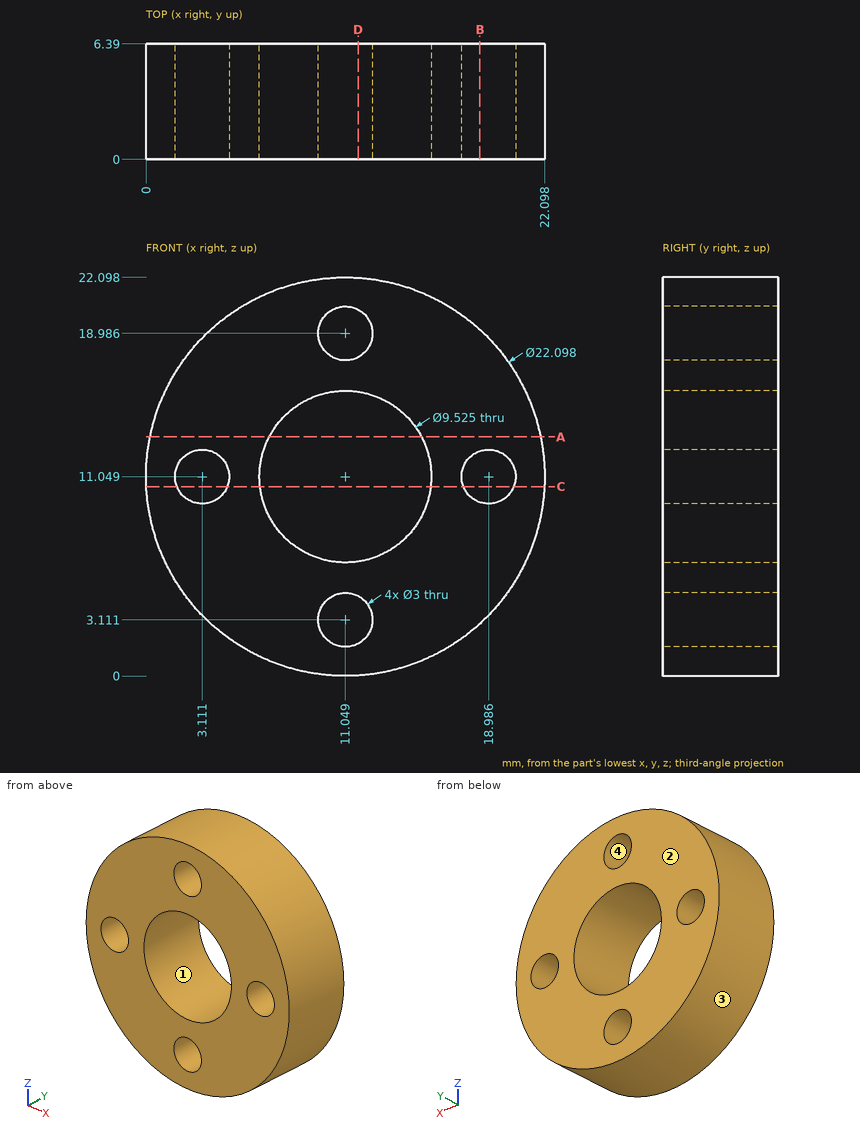
Could you check a few things on this drawing? It's one solid part, dimensions in mm from its lowest x, y, z. Coordinates: 2 decimals unless noted, no trailing zeros. Loops run counter-clockwise (first coordinate to the right, second up) from the corner with the lowest first, then second, coordinate; pieces in that order, holes last. Notation, with made-up numbers: (16.25, 85) - (43.25, 85) arc R21 cw to (43.25, 99) - close; hole circle Ø6 at (40.25, 75). An arc over 180 degrees is marked (long way). Answer as a JSON object with one key per item and string values. Group by question number.
Item 1: For pin 1 (1 mm diameter, centred on x = 15, y = 2, fed in from -Z); pin 2 (2 mm diameter, centred on x = 19, y = 1, fed in from +Z), each with a flat end and sliding along its axis, tell me the tip position at first contact or that it passes through.
Item 2: If we section it at C-C (z = 10.5): List the corners of the cut face in (x, y) for me (1 decimal).
Item 3: If we section it at A-A (z = 13.25): List the corners of the cut face in (x, y) for me (1 decimal).
Item 4: If I drill on L1, parallel to Z at x = 12.25, y = 5.75 (1 decimal); L2, parallel to X at y = 0.5, z = 9.75 (1 decimal); L3, parallel to X at y = 4.75, z = 19.75 (1 decimal), over which ranges is the centre line in solid material (lowest first)? Write a range as from..to.
Item 5: If we mould it in two halves opening along Z, with no side actions, what happens to the marked faces 1, 2, 3 and 4? For each: released by +Z, released by -Z, zero draft, split by the parting line, or undercut.
Item 6: If we section it at B-B (x = 18.5): List the corners of the cut face in (y, z) for me.
Item 7: If we section it at D-D (x = 11.75): List the corners of the cut face in (y, z) for me (1 decimal).
Returned:
{
 "1": {"pin 1": "stops at z = 0.55", "pin 2": "stops at z = 19.64"},
 "2": {"outline": "(0, 0) - (1.7, 0) - (1.7, 6.4) - (0, 6.4) - close; (4.5, 0) - (6.3, 0) - (6.3, 6.4) - (4.5, 6.4) - close; (15.8, 0) - (17.6, 0) - (17.6, 6.4) - (15.8, 6.4) - close; (20.4, 0) - (22.1, 0) - (22.1, 6.4) - (20.4, 6.4) - close"},
 "3": {"outline": "(0.2, 0) - (6.8, 0) - (6.8, 6.4) - (0.2, 6.4) - close; (15.3, 0) - (21.9, 0) - (21.9, 6.4) - (15.3, 6.4) - close"},
 "4": {"L1": "z = 0.1..2.2, 4..6.4, 15.7..18.1, 19.9..22", "L2": "x = 0.1..2.4, 3.9..6.5, 15.6..18.2, 19.7..22", "L3": "x = 4.2..9.8, 12.3..17.9"},
 "5": {"face 1": "undercut", "face 2": "zero draft", "face 3": "split by the parting line", "face 4": "undercut"},
 "6": {"outline": "(0, 2.89) - (6.39, 2.89) - (6.39, 9.63) - (0, 9.63) - close; (0, 12.47) - (6.39, 12.47) - (6.39, 19.21) - (0, 19.21) - close"},
 "7": {"outline": "(0, 0) - (6.4, 0) - (6.4, 1.8) - (0, 1.8) - close; (0, 4.4) - (6.4, 4.4) - (6.4, 6.3) - (0, 6.3) - close; (0, 15.8) - (6.4, 15.8) - (6.4, 17.7) - (0, 17.7) - close; (0, 20.3) - (6.4, 20.3) - (6.4, 22.1) - (0, 22.1) - close"}
}
